Read the model definition and answer for the solid it produces. Units are mm, in the model's axes. A direction names the side the tool comes from. Round coordinates to 2 decimals unless told otherwise and drop trailing zeros. Loops run counter-clockwise (first coordinate to the right, second up) from the corner with the lowest first, then second, coordinate; pieces in that order, holes last. Notation, with made-up numbers: M 14,42 L 43,42 A23 cw 43,53 Z; hole C -1,-21 d10. An arc over 180 degrees is marked long. Answer as CSV lines item,"result".
```python
from build123d import *

# Parameters (mm, degrees)
SKETCH1_W           = 20.32
SKETCH1_H           = 26.081708108
SKETCH1_R           = 3.175
BOSS_EXTRUDE1_DEPTH = 22.098
SKETCH2_R           = 3.175
BOSS_EXTRUDE2_DEPTH = 5.588


with BuildPart() as part:
    # Sketch1 → Boss-Extrude1 (new body)
    with BuildSketch(Plane.XY):
        with Locations((-101.659894533, 115.530854428)):
            Rectangle(SKETCH1_W, SKETCH1_H)
        with Locations(Location((-104.05047074, 124, 0), (0, 0, 180))):
            Circle(SKETCH1_R, mode=Mode.SUBTRACT)
        with Locations(Location((-104.04520642, 114, 0), (0, 0, 180))):
            Circle(SKETCH1_R, mode=Mode.SUBTRACT)
    extrude(amount=BOSS_EXTRUDE1_DEPTH)

    # Sketch2 → Boss-Extrude2 (add)
    with BuildSketch(Plane(origin=(0, 102.490000374, 0), x_dir=(1, 0, 0), z_dir=(0, 1, 0))):
        Polygon((-93.832652136, -66.597718767), (-13.072372895, -36.5640681), (-21.925888481, -12.757025827), (-64.594900087, -28.625051556), (-78.760525025, 9.46621608), (-116.851792661, -4.699408859), align=None)
        with Locations(Location((-81.347326341, -54.659995843, 0), (0, 0, 270))):
            Circle(SKETCH2_R, mode=Mode.SUBTRACT)
        with Locations(Location((-26.172504674, -33.862735355, 0), (0, 0, 270))):
            Circle(SKETCH2_R, mode=Mode.SUBTRACT)
    extrude(amount=-BOSS_EXTRUDE2_DEPTH)


solid = part.part
```
1) Find section C-C, the plane x = -99. Give the vertices of the cut face in (y, z), then the cut area to 3 significant figures.
Evaluation:
outline,"M 96.9,-1.94 L 102.49,-1.94 L 102.49,0 L 128.57,0 L 128.57,22.1 L 102.49,22.1 L 102.49,52.7 L 96.9,52.7 Z"
area,"882 mm^2"
2) Find section B-B, the plane z = 55.5. Give the vertices of the cut face in (x, y), then the cut area to 3 significant figures.
Evaluation:
outline,"M -97.96,96.9 L -84.41,96.9 L -84.41,102.49 L -97.96,102.49 Z; M -78.29,96.9 L -63.99,96.9 L -63.99,102.49 L -78.29,102.49 Z"
area,"156 mm^2"
3) A tool of negligible diameter and unlimited length cuts with its end or side. For faces 1 (the flat face through (-91.5, 115, 11)), 2 (the flat face through (-111.82, 115, 11)), 3 (the flat face through (-100, 116, 0)), from which of +Z, -Z, +X, -X, +Y, -Y can it reach the whole face along a straight path? Write none if from no direction.
Evaluation:
face 1,"+Z, -Z, +X, +Y"
face 2,"+Z, -Z, -X, +Y"
face 3,"-Z, +X, -X, +Y"
4) Determine the mould class of faces 4 (the cylindrical face through (-105.75, 111.32, 10.89)), 5 (the flat face through (-54.02, 99.74, 51.79)), 6 (the flat face through (-113, 102.49, 9)) for opening direction X: released by +X, released by -X, zero draft, split by the parting line, or undercut.
Evaluation:
face 4,"undercut"
face 5,"released by +X"
face 6,"zero draft"
5) Find section A-A, the plane y = 124. Give the vertices of the cut face in (x, z).
Evaluation:
outline,"M -111.82,0 L -107.23,0 L -107.23,22.1 L -111.82,22.1 Z; M -100.88,0 L -91.5,0 L -91.5,22.1 L -100.88,22.1 Z"
6) Straight lines are drawn through the part: line 1 (X direction, y = 114, z = 15); line 2 (X direction, y = 110, z = 19.5); line 3 (Y direction, x = -67, z = 29.5). For each, find the intervals that lie inside material, in ascending order.
Evaluation:
line 1,"x = -111.82 to -107.22, -100.87 to -91.5"
line 2,"x = -111.82 to -91.5"
line 3,"y = 96.9 to 102.49"
7) Each of these flat-tipped pins is pushed along its axis until it touches: P1, Ø10, axis at x = -104.05, y = 124, coming from the -Z side; P2, Ø8.5, axis at x = -81.35, z = 54.66, coming from the +Y side; P3, Ø0.8, axis at x = -109.5, z = 1.5, coming from the -Y side; P4, Ø10, axis at y = 105.5, z = 2, coming from the -X side. Where does it stop, or does it pass through?
Evaluation:
P1,"stops at z = 0"
P2,"stops at y = 102.49"
P3,"stops at y = 102.49"
P4,"stops at x = -116.85"
8) Find section D-D, the plane y = 106.5. Give the vertices of the cut face in (x, z), then the cut area to 3 significant figures.
Evaluation:
outline,"M -111.82,0 L -91.5,0 L -91.5,22.1 L -111.82,22.1 Z"
area,"449 mm^2"
